```python
from build123d import *

# Parameters (mm, degrees)
SALIENTE_EXTRUIR1_DEPTH = 29.5
CORTAR_EXTRUIR11_DEPTH  = 18.7
CROQUIS12_W             = 20
CROQUIS12_H             = 28.5
SALIENTE_EXTRUIR2_DEPTH = 15.5
CROQUIS6_R              = 8.5
CORTAR_EXTRUIR1_DEPTH   = 10
CROQUIS7_R              = 4.1
CORTAR_EXTRUIR2_DEPTH   = 13.5
CROQUIS8_R              = 4.4
CORTAR_EXTRUIR3_DEPTH   = 6
CROQUIS2_R              = 6.1
CORTAR_EXTRUIR4_DEPTH   = 20
CROQUIS3_R              = 6.1
CORTAR_EXTRUIR5_DEPTH   = 20
CROQUIS4_R              = 6.1
CORTAR_EXTRUIR6_DEPTH   = 20
CROQUIS5_R              = 6.1
CORTAR_EXTRUIR7_DEPTH   = 20
CORTAR_EXTRUIR8_REACH   = 35.067
CROQUIS9_R              = 3.5
CORTAR_EXTRUIR9_REACH   = 33.068
CROQUIS10_R             = 3.5
CROQUIS13_W             = 20
CROQUIS13_H             = 24.5
CORTAR_EXTRUIR10_DEPTH  = 12.5
CORTAR_EXTRUIR12_START  = -10
CROQUIS18_R             = 1.5
CORTAR_EXTRUIR12_DEPTH  = 10
CROQUIS19_R             = 1
CORTAR_EXTRUIR13_DEPTH  = 10
CROQUIS20_R             = 2.1
CORTAR_EXTRUIR14_DEPTH  = 10
CROQUIS21_R             = 5
CORTAR_EXTRUIR15_DEPTH  = 50
CROQUIS23_W             = 16.524922623
CROQUIS23_H             = 14.423778161
CORTAR_EXTRUIR16_DEPTH  = 50
REDONDEO1_R             = 4
REDONDEO2_R             = 5
REDONDEO3_R             = 4


with BuildPart() as part:
    # Croquis1 → Saliente-Extruir1 (new body)
    with BuildSketch(Plane.XY):
        with BuildLine():
            Line((5.532260486, 11.858052865), (4.932758535, 18.779017183))
            Line((4.932758535, 18.779017183), (4.932758535, 36))
            ThreePointArc((4.932758535, 36), (10.243586381, 47.979347327), (21.538526154, 54.62268913))
            Line((21.538526154, 54.62268913), (23.932758535, 55))
            Line((23.932758535, 55), (56, 55))
            ThreePointArc((56, 55), (57.424264069, 54.424264069), (58, 53))
            Line((58, 53), (58, 21.932758535))
            ThreePointArc((58, 21.932758535), (50.913097547, 9.695983483), (38, 3.932758535))
            Line((38, 3.932758535), (16.641947135, 3.932758535))
            Line((16.641947135, 3.932758535), (14.26534365, 4.78116089))
            Line((14.26534365, 4.78116089), (11.904731608, 5.153727551))
            Line((11.904731608, 5.153727551), (9.720982817, 6.124570664))
            Line((9.720982817, 6.124570664), (10.875746205, 8.011278565))
            ThreePointArc((10.875746205, 8.011278565), (20.155175368, 18.125408047), (7.690637501, 12.377476547))
            Line((7.690637501, 12.377476547), (5.532260486, 11.858052865))
        make_face()
    extrude(amount=-SALIENTE_EXTRUIR1_DEPTH)

    # Croquis15 → Cortar-Extruir11 (cut)
    with BuildSketch(Plane.XY):
        with BuildLine():
            Line((58, 42.430465887), (58, 53))
            ThreePointArc((58, 53), (57.424264069, 54.424264069), (56, 55))
            Line((56, 55), (45, 55))
            Line((45, 55), (45, 54.927917446))
            ThreePointArc((45, 54.927917446), (51.043733212, 52.876346468), (54.589631863, 47.569534113))
            Line((54.589631863, 47.569534113), (58, 42.430465887))
        make_face()
    extrude(amount=-CORTAR_EXTRUIR11_DEPTH, mode=Mode.SUBTRACT)

    # Croquis12 → Saliente-Extruir2 (add)
    with BuildSketch(Plane(origin=(0, 0, -29.5), x_dir=(-1, 0, 0), z_dir=(0, 0, -1))):
        with Locations((-48, 18.25)):
            Rectangle(CROQUIS12_W, CROQUIS12_H)
    extrude(amount=-SALIENTE_EXTRUIR2_DEPTH)

    # Croquis6 → Cortar-Extruir1 (cut)
    with BuildSketch(Plane(origin=(0, 0, -29.5), x_dir=(-1, 0, 0), z_dir=(0, 0, -1))):
        with Locations((-45, 45)):
            Circle(CROQUIS6_R)
    extrude(amount=-CORTAR_EXTRUIR1_DEPTH, mode=Mode.SUBTRACT)

    # Croquis7 → Cortar-Extruir2 (cut)
    with BuildSketch(Plane(origin=(0, 0, -19.5), x_dir=(-1, 0, 0), z_dir=(0, 0, -1))):
        with Locations((-45, 45)):
            Circle(CROQUIS7_R)
    extrude(amount=-CORTAR_EXTRUIR2_DEPTH, mode=Mode.SUBTRACT)

    # Croquis8 → Cortar-Extruir3 (cut)
    with BuildSketch(Plane.XY):
        with Locations((45, 45)):
            Circle(CROQUIS8_R)
    extrude(amount=-CORTAR_EXTRUIR3_DEPTH, mode=Mode.SUBTRACT)

    # Croquis2 → Cortar-Extruir4 (cut)
    with BuildSketch(Plane.XZ.offset(-3.932758535)):
        with Locations((30, -17.5)):
            Circle(CROQUIS2_R)
    extrude(amount=-CORTAR_EXTRUIR4_DEPTH, mode=Mode.SUBTRACT)

    # Croquis3 → Cortar-Extruir5 (cut)
    with BuildSketch(Plane(origin=(0, 55, 0), x_dir=(1, 0, 0), z_dir=(0, 1, 0))):
        with Locations((30, 17.5)):
            Circle(CROQUIS3_R)
    extrude(amount=-CORTAR_EXTRUIR5_DEPTH, mode=Mode.SUBTRACT)

    # Croquis4 → Cortar-Extruir6 (cut)
    with BuildSketch(Plane.ZY.offset(-4.932758535)):
        with Locations((-8.5, 30)):
            Circle(CROQUIS4_R)
    extrude(amount=-CORTAR_EXTRUIR6_DEPTH, mode=Mode.SUBTRACT)

    # Croquis5 → Cortar-Extruir7 (cut)
    with BuildSketch(Plane(origin=(58, 0, 0), x_dir=(0, 0, -1), z_dir=(1, 0, 0))):
        with Locations((8.5, 30)):
            Circle(CROQUIS5_R)
    extrude(amount=-CORTAR_EXTRUIR7_DEPTH, mode=Mode.SUBTRACT)

    # Croquis9 → Cortar-Extruir8 (cut, up to next)
    with BuildSketch(Plane(origin=(38, 0, 0), x_dir=(0, 0, -1), z_dir=(1, 0, 0)), mode=Mode.PRIVATE) as cortar_extruir8_sk1:
        with Locations((8.5, 30)):
            Circle(CROQUIS9_R)
    cortar_extruir8_tool1 = extrude(cortar_extruir8_sk1.sketch, amount=-CORTAR_EXTRUIR8_REACH, mode=Mode.PRIVATE) & part.part
    add(cortar_extruir8_tool1.solids().sort_by_distance((38, 30, -8.5))[0], mode=Mode.SUBTRACT)

    # Croquis10 → Cortar-Extruir9 (cut, up to next)
    with BuildSketch(Plane.XZ.offset(-23.932758535), mode=Mode.PRIVATE) as cortar_extruir9_sk1:
        with Locations((30, -17.5)):
            Circle(CROQUIS10_R)
    cortar_extruir9_tool1 = extrude(cortar_extruir9_sk1.sketch, amount=-CORTAR_EXTRUIR9_REACH, mode=Mode.PRIVATE) & part.part
    add(cortar_extruir9_tool1.solids().sort_by_distance((30, 23.932759, -17.5))[0], mode=Mode.SUBTRACT)

    # Croquis13 → Cortar-Extruir10 (cut)
    with BuildSketch(Plane(origin=(0, 0, -29.5), x_dir=(-1, 0, 0), z_dir=(0, 0, -1))):
        with Locations((-48, 20.25)):
            Rectangle(CROQUIS13_W, CROQUIS13_H)
    extrude(amount=-CORTAR_EXTRUIR10_DEPTH, mode=Mode.SUBTRACT)

    # Croquis18 → Cortar-Extruir12 (cut)
    with BuildSketch(Plane(origin=(0, 55, 0), x_dir=(1, 0, 0), z_dir=(0, 1, 0)).offset(CORTAR_EXTRUIR12_START)):
        with Locations((38.000000773, 25.50000943)):
            Circle(CROQUIS18_R)
        with Locations((52.000000773, 25.50000943)):
            Circle(CROQUIS18_R)
    extrude(amount=CORTAR_EXTRUIR12_DEPTH, mode=Mode.SUBTRACT)

    # Croquis19 → Cortar-Extruir13 (cut)
    with BuildSketch(Plane(origin=(58, 0, 0), x_dir=(0, 0, -1), z_dir=(1, 0, 0))):
        with Locations((23.5, 34)):
            Circle(CROQUIS19_R)
        with Locations((23.5, 6.5)):
            Circle(CROQUIS19_R)
    extrude(amount=-CORTAR_EXTRUIR13_DEPTH, mode=Mode.SUBTRACT)

    # Croquis20 → Cortar-Extruir14 (cut)
    with BuildSketch(Plane(origin=(0, 0, -29.5), x_dir=(-1, 0, 0), z_dir=(0, 0, -1))):
        with Locations((-16, 36)):
            Circle(CROQUIS20_R)
    extrude(amount=-CORTAR_EXTRUIR14_DEPTH, mode=Mode.SUBTRACT)

    # Croquis21 → Cortar-Extruir15 (cut)
    with BuildSketch(Plane.XY):
        with Locations((45, 45)):
            Circle(CROQUIS21_R)
    extrude(amount=-CORTAR_EXTRUIR15_DEPTH, mode=Mode.SUBTRACT)

    # Croquis23 → Cortar-Extruir16 (cut)
    with BuildSketch(Plane.XY):
        with Locations((10.637538689, 48.311889081)):
            Rectangle(CROQUIS23_W, CROQUIS23_H)
    extrude(amount=-CORTAR_EXTRUIR16_DEPTH, mode=Mode.SUBTRACT)

    # Redondeo1
    redondeo1_edges = [part.edges().sort_by_distance(p)[0] for p in [
        (6.121220744, 41.1, -14.75),
        (18.9, 53.849676427, -14.75),
    ]]
    fillet(redondeo1_edges, radius=REDONDEO1_R)

    # Redondeo2
    redondeo2_edges = [part.edges().sort_by_distance(p)[0] for p in [
        (18.9, 41.1, -14.75),
    ]]
    fillet(redondeo2_edges, radius=REDONDEO2_R)

    # Redondeo3
    redondeo3_edges = [part.edges().sort_by_distance(p)[0] for p in [
        (40, 45, 0),
    ]]
    fillet(redondeo3_edges, radius=REDONDEO3_R)


solid = part.part
```
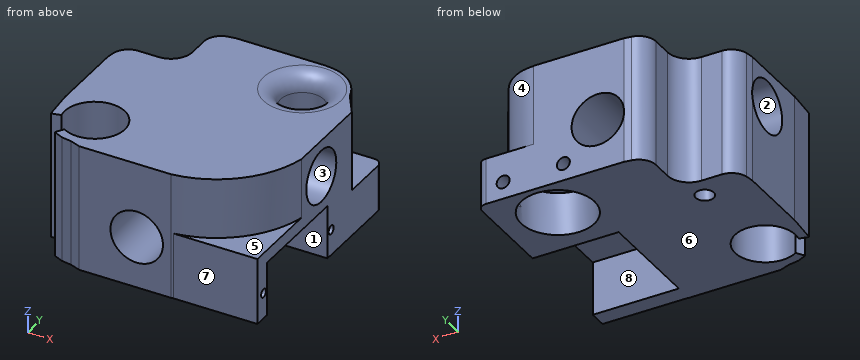
Design review of the part built by this model. Coordinates are the model's own, in mm. Face numbers are marked on the shaded views. A direction names the side the tool comes from. Give positions to 0.01 mm unless a question says otherwise; leave off trailing zeros. Loops run counter-clockwise (first coordinate to the right, second up) from the corner with the lowest first, then second, coordinate; pieces in that order, holes last. Notation, with made-up numbers: (14, 28) -> (22, 28) arc R19 ccw to (22, 45) -> close; hole circle Ø8 at (89.25, -27.75). An arc over 180 degrees is marked (long way). One line per item, written item: value.
Q1. We need section D-D on y = 18. Give the boundary of the cut face in (x, z), and give its area (3 significant figures).
Numbers:
outline: (5, -29.5) -> (8.76, -29.5) -> (8.76, 0) -> (5, 0) -> close; (20.24, -29.5) -> (38, -29.5) -> (38, -17) -> (58, -17) -> (58, -14) -> (56.78, -14) -> (56.78, 0) -> (20.24, 0) -> close; hole circle Ø12.2 at (30, -17.5)
area: 841 mm^2
Q2. We need section A-A on y = 30. Give the boundary of the cut face in (x, z), and give its area (3 significant figures).
Numbers:
outline: (4.93, -29.5) -> (38, -29.5) -> (38, -17) -> (58, -17) -> (58, -14.6) -> (38, -14.6) -> (38, -12) -> (24.93, -12) -> (24.93, -14.6) -> (4.93, -14.6) -> close; (4.93, -2.4) -> (24.93, -2.4) -> (24.93, -5) -> (38, -5) -> (38, -2.4) -> (58, -2.4) -> (58, 0) -> (4.93, 0) -> close; hole circle Ø7 at (30, -17.5)
area: 698 mm^2
Q3. Draft analysis for pull direction Y (two halves, no side actions). For the marked faces 6, 7 and 8, state which applies: pulls with the +Y half, pulls with the -Y half, needs draft (parallel to the pull), parting line crosses it, or undercut.
Numbers:
face 6: needs draft
face 7: pulls with the -Y half
face 8: undercut
Q4. For pin 1 Ø12.5 at (x, y) = (14.5, 14) entering from +Z; pin 2 Ø3.5 at (y, z) = (30.5, -6.5) entering from -X; pin 3 Ø1.4 at (x, z) = (12.5, -15.5) entering from +Y; pin 4 Ø8 at (x, y) = (39, 49) entering from -Z, all flat-tipped, find the tip position at first contact; note any pin that passes through.
Numbers:
pin 1: passes through
pin 2: stops at x = 24.93
pin 3: stops at y = 41.1
pin 4: stops at z = -29.5
Q5. We need section B-B on x = 52. Give the number of separate pieces and of enclosed holes in the cut face, and give its area (3 significant figures).
Numbers:
separate pieces: 2
enclosed holes: 3
area: 810 mm^2
Q6. For L1, parallel to Z at x = 30, y = 44; L2, parallel to Y at x = 45, z = -24.5; L3, parallel to X at y = 16, z = -18.75, list the stretches that pass through material, from the lowest coordinate up.
Numbers:
L1: z = -29.5 to -23.6, -11.4 to 0
L2: y = 4 to 8, 32.5 to 36.5, 53.5 to 55
L3: x = 5.17 to 7.79, 21.21 to 24.03, 35.97 to 38
Q7. Machinability: for the marked faces 1, 2, 3, 4 and 5, which of the approach directions +Z, -Z, +X, -X, +Y, -Y give a long, thin tool a straight path to every point of the face, cutting with its end or side? Answer none if there is none.
Numbers:
face 1: -Z, +X
face 2: -X
face 3: +X
face 4: +Z, +X, +Y
face 5: +Z, +X, -Y
